Source: CAD feature listing. Evaluate the final solid. Frame: model axes, mm. Face numbers are marked on the shaded views. Coordinates: 2 decimals unless noted, no trailing zeros. Order: outer loops, then holes, each group sorted by start corner. A loop starts at its lowest first (then second) coordinate and runs counter-clockwise, first axis right, second up. Notation, with made-up numbers: (-9, -13) -> (-4, -13) arc R25 ccw to (-4, 11) -> close; hole circle Ø7 at (11, -26.5). An arc over 180 degrees is marked (long way). Put each result on its own line as item: value.
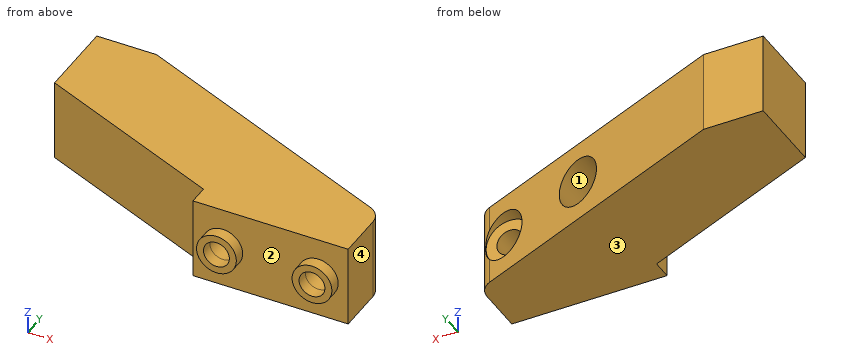
from build123d import *

# Parameters (mm, degrees)
BOSS_EXTRUDE1_DEPTH     = 20.5
CUT_EXTRUDE1_DEPTH      = 98.924715981
CUT_EXTRUDE1_DEPTH_BACK = 10
SKETCH2_R               = 3.3
SKETCH3_R               = 6
CUT_EXTRUDE2_DEPTH      = 30
SKETCH4_R               = 5
SKETCH4_R_2             = 3.25
BOSS_EXTRUDE2_DEPTH     = 3


with BuildPart() as part:
    # Sketch1 → Boss-Extrude1 (new body)
    with BuildSketch(Plane.XY):
        with BuildLine():
            Line((0, 0), (0, 6.666666667))
            ThreePointArc((0, 6.666666667), (-0.839748528, 9.440167648), (-3.076923077, 11.282051282))
            Line((-3.076923077, 11.282051282), (-72, 40))
            Line((-72, 40), (-87, 40))
            Line((-87, 40), (-87, 20))
            Line((-87, 20), (-39, 0))
            Line((-39, 0), (-39, -5))
            Line((-39, -5), (0, -5))
            Line((0, -5), (0, 0))
        make_face()
    extrude(amount=BOSS_EXTRUDE1_DEPTH)

    # Sketch2 → Cut-Extrude1 (cut, two sides: drawn at the far end of the back side and taken through both)
    with BuildSketch(Plane(origin=(0, 0, 0), x_dir=(1, 0, 0), z_dir=(0, 1, 0)).offset(-CUT_EXTRUDE1_DEPTH_BACK)):
        with Locations(Location((-7.5, -10.25, 0), (0, 0, 270))):
            Circle(SKETCH2_R)
        with Locations(Location((-31.5, -10.25, 0), (0, 0, 270))):
            Circle(SKETCH2_R)
    extrude(amount=CUT_EXTRUDE1_DEPTH + CUT_EXTRUDE1_DEPTH_BACK, mode=Mode.SUBTRACT)

    # Sketch3 → Cut-Extrude2 (cut)
    with BuildSketch(Plane(origin=(0, 40, 0), x_dir=(1, 0, 0), z_dir=(0, 1, 0))):
        with Locations(Location((-7.5, -10.25, 0), (0, 0, 270))):
            Circle(SKETCH3_R)
        with Locations(Location((-31.5, -10.25, 0), (0, 0, 270))):
            Circle(SKETCH3_R)
    extrude(amount=-CUT_EXTRUDE2_DEPTH, mode=Mode.SUBTRACT)

    # Sketch4 → Boss-Extrude2 (add)
    # profile 1 of 2: a face of its own
    with BuildSketch(Plane.XZ.offset(5)):
        with Locations(Location((-31.5, 10.25, 0), (0, 0, 90))):
            Circle(SKETCH4_R)
        with Locations(Location((-31.5, 10.25, 0), (0, 0, 270))):
            Circle(SKETCH4_R_2, mode=Mode.SUBTRACT)
    # profile 2 of 2: a face of its own
    with BuildSketch(Plane.XZ.offset(5)):
        with Locations(Location((-7.5, 10.25, 0), (0, 0, 90))):
            Circle(SKETCH4_R)
        with Locations(Location((-7.5, 10.25, 0), (0, 0, 270))):
            Circle(SKETCH4_R_2, mode=Mode.SUBTRACT)
    extrude(amount=BOSS_EXTRUDE2_DEPTH)


solid = part.part
1. Cut plane A-A on x = -6.5. Output: boundary loops of the cut face in (y, z), plus the area to 3 significant figures.
Numbers:
outline: (-8, 5.35) -> (-5, 5.35) -> (-5, 0) -> (12.71, 0) -> (12.71, 4.33) -> (10, 4.33) -> (10, 7.11) -> (-5, 7.11) -> (-5, 7.16) -> (-8, 7.16) -> close; (-8, 13.34) -> (-5, 13.34) -> (-5, 13.39) -> (10, 13.39) -> (10, 16.17) -> (12.71, 16.17) -> (12.71, 20.5) -> (-5, 20.5) -> (-5, 15.15) -> (-8, 15.15) -> close
area: 247 mm2
2. First-contact query: pin 1 (10 mm diameter, centred on x = -55, z = 2.5, fed in from +Y); pin 2 (5 mm diameter, centred on x = -7.5, z = 10.25, fed in from +Y); pin 3 (6 mm diameter, centred on x = -8, z = 13, fed in from +Y); pin 4 (1.5 mm diameter, centred on x = -42.5, z = 13, fed in from +Y). Flat tips, straight axial feed; report the tip coordinate or a pass-through.
Numbers:
pin 1: stops at y = 35
pin 2: passes through
pin 3: stops at y = 10
pin 4: stops at y = 28.02
3. Cut plane B-B on y = 33. Output: boundary loops of the cut face in (x, z), plus the area to 3 significant figures.
Numbers:
outline: (-87, 0) -> (-55.2, 0) -> (-55.2, 20.5) -> (-87, 20.5) -> close
area: 652 mm2
4. Cut plane D-D on x = -31.5. Output: boundary loops of the cut face in (y, z) (3 decimals).
Numbers:
outline: (-8, 5.25) -> (-5, 5.25) -> (-5, 0) -> (23.125, 0) -> (23.125, 4.25) -> (10, 4.25) -> (10, 6.95) -> (-5, 6.95) -> (-5, 7) -> (-8, 7) -> close; (-8, 13.5) -> (-5, 13.5) -> (-5, 13.55) -> (10, 13.55) -> (10, 16.25) -> (23.125, 16.25) -> (23.125, 20.5) -> (-5, 20.5) -> (-5, 15.25) -> (-8, 15.25) -> close
5. Ray query, line 1 along X through (y, z) = (-5.75, 10.25); line 2 along X through (y, z) = (-1.5, 10.25); line 3 along Z through (x, y) = (-7, 11). Return the intervals inside material, ascending.
Numbers:
line 1: x = -36.5 to -34.75, -28.25 to -26.5, -12.5 to -10.75, -4.25 to -2.5
line 2: x = -39 to -34.8, -28.2 to -10.8, -4.2 to 0
line 3: z = 0 to 4.27, 16.23 to 20.5
6. Cut plane C-C on z = 8.75. Count the separate pieces of the cut face and the enclosed holes in it, plus the area to 3 significant figures.
Numbers:
separate pieces: 3
enclosed holes: 0
area: 1,770 mm2
7. Pull-direction query (X, two-part tool) for the marked faces 1, 2, 3 and 4; classes: pulls with the +X half, pulls with the -X half, needs draft (parallel to the pull), parting line crosses it, or undercut.
Numbers:
face 1: undercut
face 2: undercut
face 3: needs draft
face 4: pulls with the +X half
